Model file for the job. Use its own axes, mm. A direction names the side the tool comes from. Coordinates: 2 decimals unless noted, no trailing zeros. Write each loop counter-clockwise with the first axis right and the second up, starting at its lowest first coordinate (ties: lowest second). Pieces come first, ordered by that corner, then holes.
Q1. Pin check, flat tips, straight feed: P1, Ø2, axis at y = -0.5, z = -13.5, coming from the -X side; P2, Ø1, axis at y = -2, z = 12.5, coming from the -X side; P3, Ø10, axis at x = 0, z = 0, coming from the +Y side. Stop position of each tip, or through.
Q2. Band-saw the part on D-D, the plane x = 0. Write the cut outline in (y, z), plus the area to 3 significant figures.
Q3. Which spindle directions (+Z, -Z, +X, -X, +Y, -Y) get a long thin tool onto all of the face, cutting with end or side? Do faces 1 (the cylindrical face through (31.5, 1.1, -0.2)), 2 (the flat face through (0, 0, 0)). Say none if no direction does.
Q4. Pull direction X, two halves, no side cores. Call faces 3 (the cylindrical face through (3.47, -3.49, 15.62)), 4 (the cylindrical face through (-8.054, 1.134, -1.788)), 5 (the cylindrical face through (34.12, 1.13, 18.63)): released by +X, released by -X, zero draft, split by the parting line, or undercut.
Q5. Band-saw the part on B-B, the plane y = 1. Write the cut outline in (x, z), plus the area to 3 significant figures.
Q6. Drill centre lines: probe 1 along X at (y, z) = (2, 11.5); probe 2 along X at (y, z) = (0.8, 0); probe 3 along Z at (x, y) = (-29.5, 0.75). Where is each one in solid material? Low to high.
Q7. Band-saw the part on A-A, the plane x = 28. Write the cut outline in (y, z).
Q8. Band-saw the part on C-C, the plane z = 0. Write the cut outline in (x, y), plus the area to 3 significant figures.
from build123d import *

# Parameters (mm, degrees)
SKETCH_2_R      = 3.15
SKETCH_2_R_2    = 8.25
EXTRUDE_1_DEPTH = 2.3


with BuildPart() as part:
    # ｽｹｯﾁ2 → ﾎﾞｽ - 押し出し1 (new body)
    with BuildSketch(Plane(origin=(0, 0, 0), x_dir=(1, 0, 0), z_dir=(0, 1, 0))):
        with BuildLine():
            Line((-29, 21.5), (29, 21.5))
            ThreePointArc((29, 21.5), (34.072933408, 18.703957965), (34.417821799, 12.921782213))
            ThreePointArc((34.417821799, 12.921782213), (31.500000042, 0), (34.417821799, -12.921782213))
            ThreePointArc((34.417821799, -12.921782213), (34.072933408, -18.703957965), (29, -21.5))
            Line((29, -21.5), (-29, -21.5))
            ThreePointArc((-29, -21.5), (-34.072933408, -18.703957965), (-34.417821799, -12.921782213))
            ThreePointArc((-34.417821799, -12.921782213), (-31.499999945, 0), (-34.417821799, 12.921782213))
            ThreePointArc((-34.417821799, 12.921782213), (-34.072933408, 18.703957965), (-29, 21.5))
        make_face()
        with Locations(Location((28, 14, 0), (0, 0, 270))):
            Circle(SKETCH_2_R, mode=Mode.SUBTRACT)
        with Locations(Location((28, -14, 0), (0, 0, 270))):
            Circle(SKETCH_2_R, mode=Mode.SUBTRACT)
        with Locations(Location((-28, 14, 0), (0, 0, 270))):
            Circle(SKETCH_2_R, mode=Mode.SUBTRACT)
        with Locations(Location((-28, -14, 0), (0, 0, 270))):
            Circle(SKETCH_2_R, mode=Mode.SUBTRACT)
        with Locations(Location((0, 0, 0), (0, 0, 270))):
            Circle(SKETCH_2_R_2, mode=Mode.SUBTRACT)
    extrude(amount=EXTRUDE_1_DEPTH)

    # ｽｹｯﾁ4 → 回転1 (revolve)
    with BuildSketch(Plane.XY, mode=Mode.PRIVATE) as revolve_1_sk:
        with BuildLine():
            Line((13, 0), (0, 0))
            Line((0, 0), (0, -4))
            Line((0, -4), (16, -4))
            Line((16, -4), (16, -3))
            ThreePointArc((16, -3), (15.121320344, -0.878679656), (13, 0))
        make_face()
    revolve(revolve_1_sk.sketch.rotate(Axis((0, 0, 0), (0, -1, 0)), 180), axis=Axis((0, 0, 0), (0, -1, 0)))


solid = part.part
Answer sheet:
1. P1: stops at x = -34.89
1. P2: stops at x = -10.37
1. P3: stops at y = 0
2. outline: (-4, -16) - (-3, -16) arc R3 ccw to (0, -13) - (0, -21.5) - (2.3, -21.5) - (2.3, -8.25) - (0, -8.25) - (0, 8.25) - (2.3, 8.25) - (2.3, 21.5) - (0, 21.5) - (0, 13) arc R3 ccw to (-3, 16) - (-4, 16) - close
2. area: 185 mm2
3. face 1: +X, +Y, -Y
3. face 2: +Y
4. face 3: split by the parting line
4. face 4: undercut
4. face 5: released by +X
5. outline: (-34.42, -12.92) arc R6 ccw to (-29, -21.5) - (29, -21.5) arc R6 ccw to (34.42, -12.92) arc R30.07 cw to (34.42, 12.92) arc R6 ccw to (29, 21.5) - (-29, 21.5) arc R6 ccw to (-34.42, 12.92) arc R30.07 cw to start; hole circle Ø6.3 at (-28, -14); hole circle Ø6.3 at (-28, 14); hole circle Ø16.5 at (0, 0); hole circle Ø6.3 at (28, -14); hole circle Ø6.3 at (28, 14)
5. area: 2,510 mm2
6. probe 1: x = -33.79 to -29.92, -26.08 to 26.08, 29.92 to 33.79
6. probe 2: x = -31.5 to -8.25, 8.25 to 31.5
6. probe 3: z = -21.48 to -16.77, -11.23 to 11.23, 16.77 to 21.48
7. outline: (0, -21.5) - (2.3, -21.5) - (2.3, -17.15) - (0, -17.15) - close; (0, -10.85) - (2.3, -10.85) - (2.3, 10.85) - (0, 10.85) - close; (0, 17.15) - (2.3, 17.15) - (2.3, 21.5) - (0, 21.5) - close
8. outline: (-31.5, 0) - (-13, 0) arc R3 ccw to (-16, -3) - (-16, -4) - (16, -4) - (16, -3) arc R3 ccw to (13, 0) - (31.5, 0) - (31.5, 2.3) - (8.25, 2.3) - (8.25, 0) - (-8.25, 0) - (-8.25, 2.3) - (-31.5, 2.3) - close
8. area: 231 mm2
